```python
from build123d import *

# Parameters (mm, degrees)
SKETCH1_R           = 101.859163579
BOSS_EXTRUDE1_DEPTH = 3


with BuildPart() as part:
    # Sketch1 → Boss-Extrude1 (new body)
    with BuildSketch(Plane.XY):
        Circle(SKETCH1_R)
        with BuildLine():
            Line((-38.589791853, -13.042222407), (-73.230808005, -33.042222407))
            ThreePointArc((-73.230808005, -33.042222407), (-75.962858812, -32.3101716), (-75.230808005, -29.578120792))
            Line((-75.230808005, -29.578120792), (-40.589791853, -9.578120792))
            ThreePointArc((-40.589791853, -9.578120792), (-37.857741046, -10.3101716), (-38.589791853, -13.042222407))
        make_face(mode=Mode.SUBTRACT)
        with BuildLine():
            Line((-28.573863011, -30.544431757), (-63.282032303, -50.392304845))
            ThreePointArc((-63.282032303, -50.392304845), (-66.01408311, -49.660254038), (-65.282032303, -46.92820323))
            Line((-65.282032303, -46.92820323), (-30.739185351, -26.793983449))
            Line((-30.739185351, -26.793983449), (-30.723714344, -26.78496576))
            ThreePointArc((-30.723714344, -26.78496576), (-27.765727873, -27.577555846), (-28.558317959, -30.535542316))
            Line((-28.558317959, -30.535542316), (-28.573863011, -30.544431757))
        make_face(mode=Mode.SUBTRACT)
        with BuildLine():
            Line((-24.980762114, -16.732050808), (-57.812135025, -35.687252796))
            ThreePointArc((-57.812135025, -35.687252796), (-60.544185832, -34.955201988), (-59.812135025, -32.223151181))
            Line((-59.812135025, -32.223151181), (-26.980762114, -13.267949192))
            ThreePointArc((-26.980762114, -13.267949192), (-24.248711306, -14), (-24.980762114, -16.732050808))
        make_face(mode=Mode.SUBTRACT)
        with BuildLine():
            Line((30.589791853, -26.898628868), (65.230808005, -46.898628868))
            ThreePointArc((65.230808005, -46.898628868), (65.962858812, -49.630679675), (63.230808005, -50.362730483))
            Line((63.230808005, -50.362730483), (28.589791853, -30.362730483))
            ThreePointArc((28.589791853, -30.362730483), (27.857741046, -27.630679675), (30.589791853, -26.898628868))
        make_face(mode=Mode.SUBTRACT)
        with BuildLine():
            Line((26.980762114, -13.267949192), (59.812135025, -32.223151181))
            ThreePointArc((59.812135025, -32.223151181), (60.544185832, -34.955201988), (57.812135025, -35.687252796))
            Line((57.812135025, -35.687252796), (24.980762114, -16.732050808))
            ThreePointArc((24.980762114, -16.732050808), (24.248711306, -14), (26.980762114, -13.267949192))
        make_face(mode=Mode.SUBTRACT)
        with BuildLine():
            Line((40.739185351, -9.473475374), (75.282032303, -29.607695155))
            ThreePointArc((75.282032303, -29.607695155), (76.01408311, -32.339745962), (73.282032303, -33.07179677))
            Line((73.282032303, -33.07179677), (38.573863011, -13.223923681))
            Line((38.573863011, -13.223923681), (38.558317959, -13.21503424))
            ThreePointArc((38.558317959, -13.21503424), (37.765727873, -10.25704777), (40.723714344, -9.464457684))
            Line((40.723714344, -9.464457684), (40.739185351, -9.473475374))
        make_face(mode=Mode.SUBTRACT)
        with BuildLine():
            Line((-2, 30), (-2, 67.910403976))
            ThreePointArc((-2, 67.910403976), (0, 69.910403976), (2, 67.910403976))
            Line((2, 67.910403976), (2, 30))
            ThreePointArc((2, 30), (0, 28), (-2, 30))
        make_face(mode=Mode.SUBTRACT)
        with BuildLine():
            Line((-12.16532234, 40.01790713), (-12, 80))
            ThreePointArc((-12, 80), (-10, 82), (-8, 80))
            Line((-8, 80), (-7.83467766, 40.01790713))
            Line((-7.83467766, 40.01790713), (-7.834603616, 40))
            ThreePointArc((-7.834603616, 40), (-10, 37.834603616), (-12.165396384, 40))
            Line((-12.165396384, 40), (-12.16532234, 40.01790713))
        make_face(mode=Mode.SUBTRACT)
        with BuildLine():
            Line((8, 39.940851275), (8, 79.940851275))
            ThreePointArc((8, 79.940851275), (10, 81.940851275), (12, 79.940851275))
            Line((12, 79.940851275), (12, 39.940851275))
            ThreePointArc((12, 39.940851275), (10, 37.940851275), (8, 39.940851275))
        make_face(mode=Mode.SUBTRACT)
    extrude(amount=BOSS_EXTRUDE1_DEPTH)


solid = part.part
```
Source: CAD feature listing. Evaluate the final solid. Frame: model axes, mm. A direction names the side the tool comes from. Give positions to 0.01 mm unless a question says otherwise; leave off trailing zeros. Order: outer loops, then holes, each group sorted by start corner. A loop starts at its lowest first (then second) coordinate and runs counter-clockwise, first axis right, second up. Notation, with made-up numbers: (89, -16) -> (124, -16) arc R33 cw to (124, 16) -> close; hole circle Ø3 at (-27, 52.25). An arc over 180 degrees is marked (long way). Use a Markdown table: item, result.
Q1. Section C-C (z = 2.5). State how many separate pieces and enclosed holes the cut face has, and give its area (3 significant figures).
A:
| item | result |
|---|---|
| separate pieces | 1 |
| enclosed holes | 9 |
| area | 31,000 mm^2 |
Q2. Access query for faces 4 (the face through (-58.153, -19.718, 1.479)), 5 (the face through (-1, 1, 0)). Directions: +Z, -Z, +X, -X, +Y, -Y. A direction counts if a zero-diameter tool reaches every point of the face in a straight line with its end or side. Return the directions, or none.
A:
| item | result |
|---|---|
| face 4 | +Z, -Z |
| face 5 | -Z, +X, -X, +Y, -Y |
Q3. Section B-B (x = 50). Return the cut outline in (y, z).
A:
| item | result |
|---|---|
| outline | (-88.74, 0) -> (-42.72, 0) -> (-42.72, 3) -> (-88.74, 3) -> close; (-38.11, 0) -> (-31.18, 0) -> (-31.18, 3) -> (-38.11, 3) -> close; (-26.56, 0) -> (-19.76, 0) -> (-19.76, 3) -> (-26.56, 3) -> close; (-14.87, 0) -> (88.74, 0) -> (88.74, 3) -> (-14.87, 3) -> close |
Q4. Section A-A (y = 55.5). Return the cut outline in (x, z).
A:
| item | result |
|---|---|
| outline | (-85.41, 0) -> (-12.1, 0) -> (-12.1, 3) -> (-85.41, 3) -> close; (-7.9, 0) -> (-2, 0) -> (-2, 3) -> (-7.9, 3) -> close; (2, 0) -> (8, 0) -> (8, 3) -> (2, 3) -> close; (12, 0) -> (85.41, 0) -> (85.41, 3) -> (12, 3) -> close |
Q5. First-contact query: P1, Ø1, axis at y = 66.5, z = 1, coming from the +X side; P2, Ø6, axis at x = -23, y = 31, coming from the -Z side; P3, Ø1, axis at y = 36.5, z = 2.5, coming from the +X side. Flat tips, straight axial feed; report the tip coordinate or a pass-through.
A:
| item | result |
|---|---|
| P1 | x = 77.58 |
| P2 | z = 0 |
| P3 | x = 95.29 |
Q6. Material intervals for line 1 (Y direction, x = -60, z = 0.45); line 2 (Y direction, x = 54.5, z = 1.4) (3 decimals); line 3 (X direction, y = 0.5, z = 1.1), sorted ascending. Write a range as [from, to].
A:
| item | result |
|---|---|
| line 1 | [-82.31, -48.52], [-43.85, -35.56], [-32.35, -25.4], [-20.78, 82.31] |
| line 2 | [-86.053, -45.322], [-40.703, -33.775], [-29.156, -22.331], [-17.494, 86.053] |
| line 3 | [-101.86, 101.86] |
Q7. Section D-D (x = 88). Return the cut outline in (y, z), and give its area (3 significant figures).
A:
| item | result |
|---|---|
| outline | (-51.3, 0) -> (51.3, 0) -> (51.3, 3) -> (-51.3, 3) -> close |
| area | 308 mm^2 |
Q8. Pull-direction query (X, two-part tool) for faces 1 (the face through (-1, 1, 3)), 2 (the face through (-13.26, 100.992, 1.479)), 3 (the face through (43.167, -22.613, 1.479)); classes: +X half, -X half, draft (parallel to the pull), parting line (faces both ways), or undercut.
A:
| item | result |
|---|---|
| face 1 | draft |
| face 2 | parting line |
| face 3 | undercut |
